Autodesk Inventor part; units mm, degrees
ref_plane "YZ Plane" through (0, 0, 0) normal (1, 0, 0) x (0, 1, 0)
ref_plane "XZ Plane" through (0, 0, 0) normal (0, 1, 0) x (-1, 0, 0)
ref_plane "XY Plane" through (0, 0, 0) normal (0, 0, 1) x (1, 0, 0)
sketch "main" plane through (0, 0, 0) normal (0, 0, 1) x (1, 0, 0)
  circle A0 centre (11.6396, 18.419) radius 2.1844
  circle A1 centre (-13.7604, 18.419) radius 2.1844
  arc A2 (-13.7604, 24.769) -> (-19.6572, 16.0633) centre (-13.7604, 18.419) ccw
  arc A3 (17.9587, 17.7933) -> (11.6396, 24.769) centre (11.6396, 18.419) ccw
  line L0 (-19.6572, 16.0633) -> (0.6972, -34.8883)
  line L1 (17.9587, 17.7933) -> (12.9132, -33.1583)
  line L2 (-13.7604, 24.769) -> (11.6396, 24.769)
  circle A4 centre (6.5941, -32.5326) radius 2.0955
  arc A5 (0.6972, -34.8883) -> (12.9132, -33.1583) centre (6.5941, -32.5326) ccw
  point P0 (1.7688, 7.28)
  dimension "d0" = 12.7
  dimension "d1" = 12.7
  dimension "d2" = 12.7
  dimension "d5" = 4.191
sketch "Sketch1" plane through (0, 0, 0) normal (0, 0, 1) x (1, 0, 0)
  circle A0 centre (25.4, 0) radius 2.1844
  circle A1 centre (0, 0) radius 2.1844
  arc A2 (0, 6.35) -> (-5.8969, -2.3557) centre (0, 0) ccw
  arc A3 (31.7191, -0.6258) -> (25.4, 6.35) centre (25.4, 0) ccw
  line L0 (-5.8969, -2.3557) -> (14.4576, -53.3073)
  line L1 (31.7191, -0.6258) -> (26.6735, -51.5774)
  line L2 (0, 6.35) -> (25.4, 6.35)
  circle A4 centre (20.3545, -50.9516) radius 2.0955
  arc A5 (14.4576, -53.3073) -> (26.6735, -51.5774) centre (20.3545, -50.9516) ccw
extrude "Extrusion1" add sketch "Sketch1" along normal blind 1.5875
properties part number "vertical_wing_gusset" material "Acetal Resin, White"
For this review, take the finished solid that the model builds, in its own axes (mm). Coordinates: 2 decimals unless noted, no trailing zeros. Order: outer loops, then holes, each group sorted by start corner. A loop starts at its lowest first (then second) coordinate and runs counter-clockwise, first axis right, second up. Notation, with made-up numbers: (-38, 11) -> (21, 11) arc R21 cw to (21, 36) -> close; hole circle Ø5 at (33.5, -3). An arc over 180 degrees is marked (long way). Use CSV: the item, a comma, the result in double quotes. Start each with the question number.
Item 1: We need section B-B, the plane x = 1. Give the boundary of the cut face in (y, z).
Item 2: We need section D-D, the plane y = -8.5. Give the boundary of the cut face in (x, z).
Item 3: Draft analysis for pull direction X (two halves, no side actions). For faces 1 (the face through (17, -18, 0)), 2 (the face through (21.36, -57.22, 0.78)), 3 (the face through (27.418, 0.837, 0.783)), 4 (the face through (21.32, -49.09, 0.78)), state which applies: pulls with the +X half, pulls with the -X half, needs draft (parallel to the pull), parting line crosses it, or undercut.
Item 4: Insertion check: pin 1 (2.5 mm diameter, centred on x = 25.4, y = 0, fed in from +Z). The pin has a flat end and moves straight along its axis. Give the tip position at first contact, or say it passes through.
Item 5: We need section A-A, the plane y = 0. Give the boundary of the cut face in (x, z), then the cut area to 3 significant figures.
Item 6: Wall thickness on probe 1 along X at (y, z) = (1, 1); probe 2 along X at (y, z) = (-2, 0.3); probe 3 along Y at (x, z) = (20.5, 0.5): over which ranges is each line inside the solid? List them lowest first.
Item 7: We need section C-C, the plane z = 0.4. Give the boundary of the cut face in (x, y), then the cut area to 3 significant figures.
Derived:
1,outline,"(-19.62, 0) -> (-1.94, 0) -> (-1.94, 1.59) -> (-19.62, 1.59) -> close; (1.94, 0) -> (6.35, 0) -> (6.35, 1.59) -> (1.94, 1.59) -> close"
2,outline,"(-3.44, 0) -> (30.94, 0) -> (30.94, 1.59) -> (-3.44, 1.59) -> close"
3,face 1,"needs draft"
3,face 2,"parting line crosses it"
3,face 3,"undercut"
3,face 4,"undercut"
4,pin 1,"passes through"
5,outline,"(-6.35, 0) -> (-2.18, 0) -> (-2.18, 1.59) -> (-6.35, 1.59) -> close; (2.18, 0) -> (23.22, 0) -> (23.22, 1.59) -> (2.18, 1.59) -> close; (27.58, 0) -> (31.75, 0) -> (31.75, 1.59) -> (27.58, 1.59) -> close"
5,area,"46.6 mm^2"
6,probe 1,"x = -6.27 to -1.94, 1.94 to 23.46, 27.34 to 31.67"
6,probe 2,"x = -6.03 to -0.88, 0.88 to 24.52, 26.28 to 31.58"
6,probe 3,"y = -57.3 to -53.04, -48.86 to 6.35"
7,outline,"(-5.9, -2.36) -> (14.46, -53.31) arc R6.35 ccw to (26.67, -51.58) -> (31.72, -0.63) arc R6.35 ccw to (25.4, 6.35) -> (0, 6.35) arc R6.35 ccw to start; hole circle Ø4.37 at (0, 0); hole circle Ø4.19 at (20.35, -50.95); hole circle Ø4.37 at (25.4, 0)"
7,area,"1,560 mm^2"
